Source: three-view drawing plus pictorial views. Frame: mm from the lowest corner of the part. Round coordinates to 2 decimals unless told otherwise and drop trailing zeros. Loops run counter-clockwise (first coordinate to the right, second up) from the corner with the lowest first, then second, coordinate; pieces in that order, holes last. Notation, with made-up numbers: M 12,7 L 17,7 A16 cw 17,21 Z; hole C -18.5,83 d10. An arc over 180 degrees is marked long. Write each question's results on one line, items separated by ' | '.
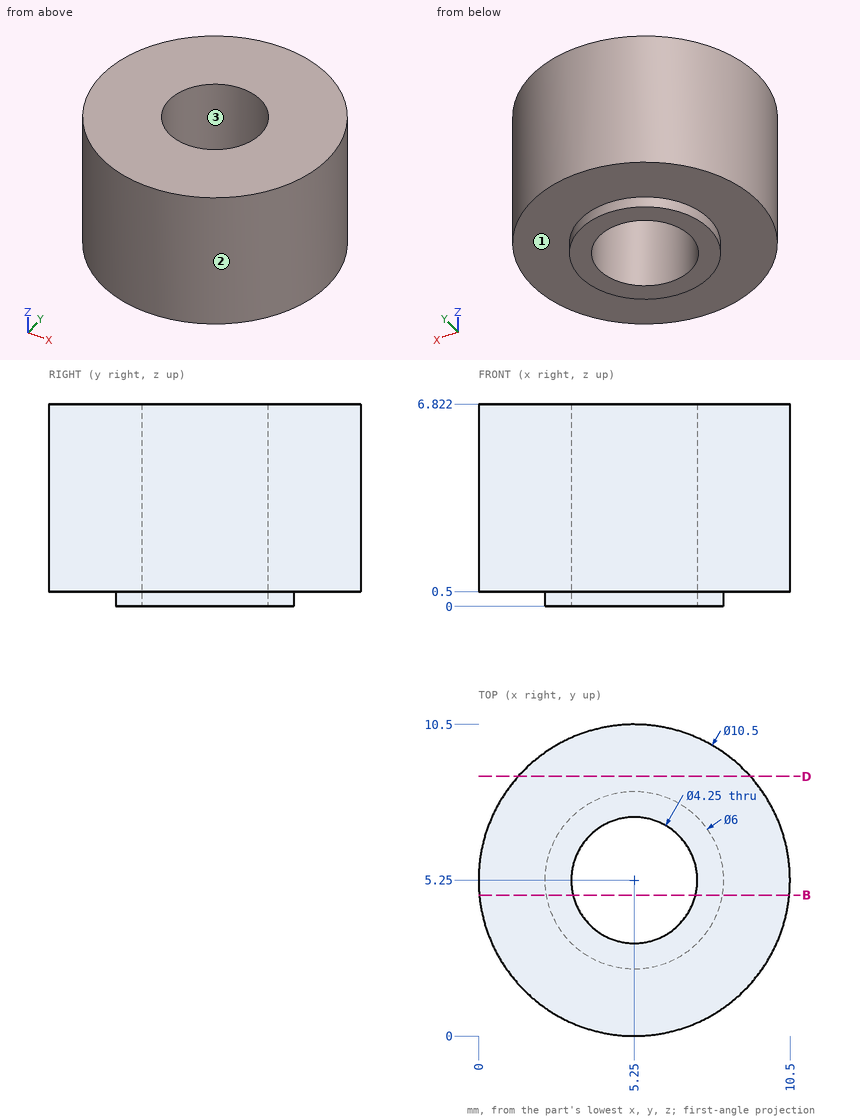
1. Section D-D (y = 8.75). Output: boundary loops of the cut face in (x, z).
Answer key:
outline: M 1.34,0.5 L 9.16,0.5 L 9.16,6.82 L 1.34,6.82 Z
2. Draft query along Y for the marked faces 1, 2 and 3. Return one class per face: pulls with the +Y half, pulls with the -Y half, needs draft (parallel to the pull), parting line crosses it, or undercut.
Answer key:
face 1: needs draft | face 2: parting line crosses it | face 3: undercut
3. Section B-B (y = 4.75). Output: boundary loops of the cut face in (x, z) (1 decimal).
Answer key:
outline: M 0,0.5 L 2.3,0.5 L 2.3,0 L 3.2,0 L 3.2,6.8 L 0,6.8 Z; M 7.3,0 L 8.2,0 L 8.2,0.5 L 10.5,0.5 L 10.5,6.8 L 7.3,6.8 Z
4. Ray query, probe 1 along Y at (x, z) = (5.25, 4.5) (1 decimal); probe 2 along Z at (x, y) = (9.75, 7); probe 3 along Y at (x, z) = (6.25, 3.25) (1 decimal). Return the intervals inside material, ascending.
Answer key:
probe 1: y = 0 to 3.1, 7.4 to 10.5 | probe 2: z = 0.5 to 6.82 | probe 3: y = 0.1 to 3.4, 7.1 to 10.4
5. Pin query (flat end, axial travel): P1, Ø1.5, axis at x = 1.5, y = 9, coming from the -Z side; P2, Ø2, axis at y = 7, z = 5.5, coming from the +X side. Return the tip coordinate at first contact, or that it passes through.
Answer key:
P1: stops at z = 0.5 | P2: stops at x = 10.45
